Source: CAD feature listing. Evaluate the final solid. Frame: model axes, mm. Face numbers are marked on the shaded views. Coordinates: 2 decimals unless noted, no trailing zeros. Order: outer loops, then holes, each group sorted by start corner. A loop starts at its lowest first (then second) coordinate and runs counter-clockwise, first axis right, second up.
```python
from build123d import *

# Parameters (mm, degrees)
F0_W     = 13.335
F0_H     = 15.7
F1_DEPTH = 20.57
F3_DEPTH = 4.3
F5_DEPTH = 13.336


with BuildPart() as f1:
    # F0 (on Front) → F1 (new body)
    with BuildSketch(Plane.XZ):
        Rectangle(F0_W, F0_H)
    extrude(amount=-F1_DEPTH)

    # F2 (on face) → F3 (join)
    with BuildSketch(Plane(origin=(0, 0, -7.85), x_dir=(1, 0, 0), z_dir=(0, 0, -1))):
        with BuildLine():
            Line((6.6675, -10.9442927568), (6.6675, -9.8757072432))
            ThreePointArc((6.6675, -9.8757072432), (3.405, -10.41), (6.6675, -10.9442927568))
        make_face()
        with BuildLine():
            ThreePointArc((-3.405, -10.41), (-4.8092949022, -8.757019737), (-6.6675, -9.8757072432))
            Line((-6.6675, -9.8757072432), (-6.6675, -10.9442927568))
            ThreePointArc((-6.6675, -10.9442927568), (-4.8092949022, -12.062980263), (-3.405, -10.41))
        make_face()
    extrude(amount=F3_DEPTH)

    # F4 (on face) → F5 (cut, through all)
    with BuildSketch(Plane.YZ.offset(6.6675)):
        with BuildLine():
            Line((18.1063264608, 4.1939658113), (20.57, -3.2797483727))
            Line((20.57, -3.2797483727), (20.57, 7.85))
            Line((20.57, 7.85), (13.3700780571, 7.85))
            add(Edge.make_bspline(
                [(18.1063264608, 4.1939658113), (16.9114023447, 7.1921413764), (16.3248032331, 7.3876748793), (13.3700780571, 7.85)],
                knots=[0, 0, 0, 0, 5.9831960466, 5.9831960466, 5.9831960466, 5.9831960466], degree=3))
        make_face()
    extrude(amount=-F5_DEPTH, mode=Mode.SUBTRACT)


solid = f1.part
```
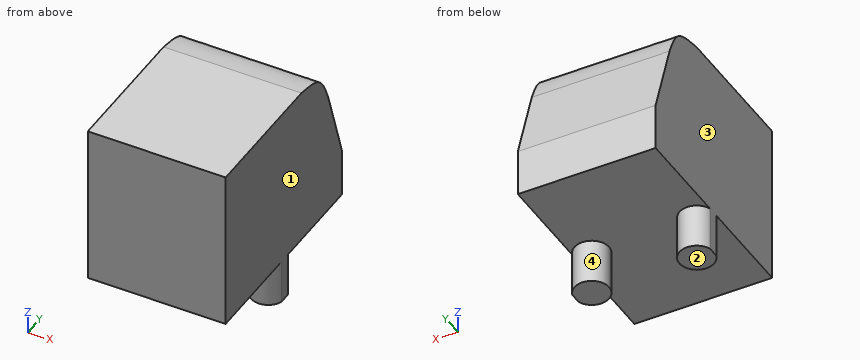
Q1. Pin query (flat end, axial travel): P1, Ø6.5, axis at x = 0, y = 9.5, coming from the -Z side; P2, Ø3, axis at x = -4.5, z = 0.5, coming from the +Y side. Return the tip coordinate at first contact, or that it passes through.
Solutions:
P1: stops at z = -7.85
P2: stops at y = 19.82
Q2. Material intervals for line 1 along Z through (x, y) = (1.5, 3.75); line 2 along Z through (x, y) = (0, 18); line 3 along Y through (x, z) = (2.5, -0.75), sorted ascending.
Solutions:
line 1: z = -7.85 to 7.85
line 2: z = -7.85 to 4.46
line 3: y = 0 to 19.74
Q3. Pull-direction query (X, two-part tool) for the marked faces 1, 2, 3 and 4; classes: pulls with the +X half, pulls with the -X half, needs draft (parallel to the pull), parting line crosses it, or undercut.
Solutions:
face 1: pulls with the +X half
face 2: needs draft
face 3: pulls with the -X half
face 4: undercut
Q4. Section query B-B on z = 1.5. Output: boundary loops of the cut face in (x, y).
Solutions:
outline: (-6.67, 0) - (6.67, 0) - (6.67, 18.99) - (-6.67, 18.99) - close
